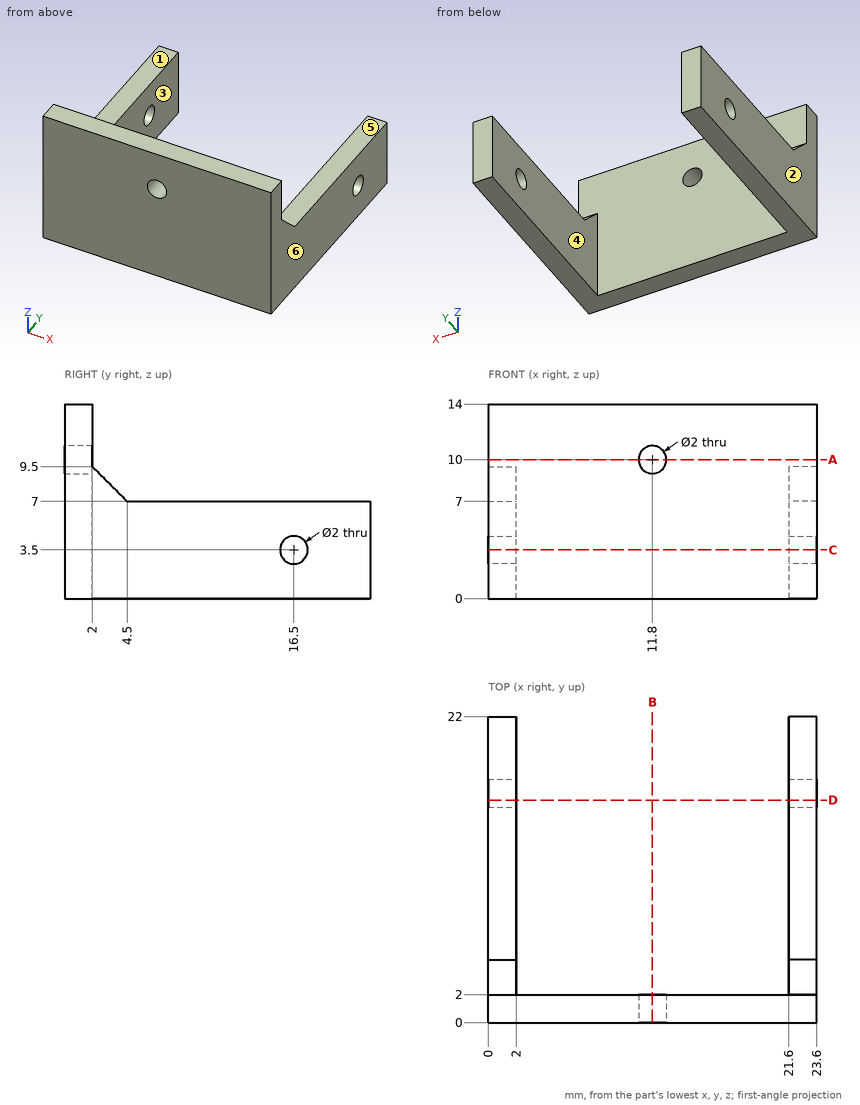
Job drawing, mm, ordinate dimensions from the low corner. One solid piece. A direction names the side the tool comes from. Give positions to 0.01 mm unless a question says otherwise; leave off trailing zeros. Order: outer loops, then holes, each group sorted by start corner. A loop starts at its lowest first (then second) coordinate and runs counter-clockwise, first axis right, second up. Notation, with made-up numbers: (46.25, -14.75) -> (72.25, -14.75) arc R23 cw to (72.25, 21.25) -> close; hole circle Ø10 at (36, 32). An arc over 180 degrees is marked (long way). Return JSON: item names as keys, results as strings.
Q1. Which spindle directions (+Z, -Z, +X, -X, +Y, -Y) get a long thin tool onto all of the face, cutting with end or side? Do the marked faces 4, 5 and 6. Say none if no direction does.
Working result:
{"face 4": "+Z, -Z, +Y", "face 5": "+Z, +X, -X, +Y", "face 6": "+Z, -Z, +X, +Y, -Y"}
Q2. Flat gauge pins, fed straight in: pin 1 (0.6 mm diameter, centred on x = 23, y = 14.5, fed in from +Z); pin 2 (8 mm diameter, centred on x = 16.5, y = 19.5, fed in from -Z). Where does each tip first touch, or does it go through?
Working result:
{"pin 1": "z = 7", "pin 2": "through"}
Q3. Drill centre lines: line 1 (X direction, y = 15, z = 1.5); line 2 (Y direction, x = 23, z = 3.5); line 3 (Y direction, x = 9, z = 10.75). Where is each one in solid material? Low to high.
Working result:
{"line 1": "0 to 2, 21.6 to 23.6", "line 2": "0 to 15.5, 17.5 to 22", "line 3": "0 to 2"}
Q4. Saw through at C-C (z = 3.5). Write the cut outline in (x, y), then the cut area to 3 significant figures.
Working result:
{"outline": "(0, 0) -> (23.6, 0) -> (23.6, 15.5) -> (21.6, 15.5) -> (21.6, 2) -> (2, 2) -> (2, 15.5) -> (0, 15.5) -> close; (0, 17.5) -> (2, 17.5) -> (2, 22) -> (0, 22) -> close; (21.6, 17.5) -> (23.6, 17.5) -> (23.6, 22) -> (21.6, 22) -> close", "area": "119 mm²"}
Q5. Saw through at D-D (y = 16). Write the cut outline in (x, z).
Working result:
{"outline": "(0, 0) -> (2, 0) -> (2, 2.63) -> (0, 2.63) -> close; (0, 4.37) -> (2, 4.37) -> (2, 7) -> (0, 7) -> close; (21.6, 0) -> (23.6, 0) -> (23.6, 2.63) -> (21.6, 2.63) -> close; (21.6, 4.37) -> (23.6, 4.37) -> (23.6, 7) -> (21.6, 7) -> close"}
Q6. Saw through at A-A (z = 10). Write the cut outline in (x, y).
Working result:
{"outline": "(0, 0) -> (10.8, 0) -> (10.8, 2) -> (0, 2) -> close; (12.8, 0) -> (23.6, 0) -> (23.6, 2) -> (12.8, 2) -> close"}
Q7. Saw through at B-B (x = 11.8). Write the cut outline in (y, z), then the cut area to 3 significant figures.
Working result:
{"outline": "(0, 0) -> (2, 0) -> (2, 9) -> (0, 9) -> close; (0, 11) -> (2, 11) -> (2, 14) -> (0, 14) -> close", "area": "24.0 mm²"}
Q8. Mould opens along X. For the marked faces 1, 2 and 3 say: pulls with the +X half, pulls with the -X half, needs draft (parallel to the pull), parting line crosses it, or undercut.
Working result:
{"face 1": "needs draft", "face 2": "pulls with the -X half", "face 3": "undercut"}
